Geometry: final body of the model. Coordinates: model frame, mm. Round coordinates to 2 decimals unless told otherwise and drop trailing zeros. Write each loop counter-clockwise with the first axis right and the second up, starting at its lowest first coordinate (ties: lowest second). Pieces come first, ordered by that corner, then holes. Notation, with made-up numbers: M -25,46 L -21,46 A18 ccw -21,54 Z; hole C -17,84.25 d1. An arc over 180 degrees is marked long. Use one line per item in the form item = value. Start each with the question number.
Item 1: Section query B-B (z = 31). Return loops of the section in (x, y).
Item 2: Ray query, probe 1 along X at (y, z) = (14, 29); probe 2 along Y at (x, z) = (131, 33); probe 3 along Y at (x, z) = (15, 29). Return the intervals inside material, ascending.
Item 3: Section query A-A (y = 15). Return loops of the section in (x, z).
Item 4: Pin query (flat end, axial travel): pin 1 Ø5 at (x, y) = (105, 76) entering from -Z; pin 2 Ø7 at (x, y) = (185, 15) entering from -Z; pin 3 Ø3 at (x, z) = (133.5, 22) entering from +Y; pin 4 Ø1 at (x, z) = (42, 5.5) entering from +Y. Return the tip coordinate at first contact, or that it passes through.
from build123d import *

# Parameters (mm, degrees)
F1_DEPTH = 50
F2_R     = 5
F3_R     = 4
F4_DEPTH = 50.001


with BuildPart() as f1:
    # F0 (on Top) → F1 (new body)
    with BuildSketch(Plane.XY):
        with BuildLine():
            Line((0, 57.2570811482), (0, 0))
            Line((0, 0), (200, 0))
            Line((200, 0), (200, 57.2570811482))
            ThreePointArc((200, 57.2570811482), (199.3836985076, 59.6619070036), (197.6867250421, 61.4738937535))
            Line((197.6867250421, 61.4738937535), (138.4492468932, 99.2168126053))
            ThreePointArc((138.4492468932, 99.2168126053), (137.1617961225, 99.8002116113), (135.7625218511, 100))
            Line((135.7625218511, 100), (129.5803989155, 100))
            ThreePointArc((129.5803989155, 100), (126.3529127937, 101.1811869209), (124.6503324296, 104.1666666667))
            ThreePointArc((124.6503324296, 104.1666666667), (100, 125), (75.3496675704, 104.1666666667))
            ThreePointArc((75.3496675704, 104.1666666667), (73.6470872063, 101.1811869209), (70.4196010845, 100))
            Line((70.4196010845, 100), (64.2374781489, 100))
            ThreePointArc((64.2374781489, 100), (62.8382038775, 99.8002116113), (61.5507531068, 99.2168126053))
            Line((61.5507531068, 99.2168126053), (2.3132749579, 61.4738937535))
            ThreePointArc((2.3132749579, 61.4738937535), (0.6163014924, 59.6619070036), (0, 57.2570811482))
        make_face()
    extrude(amount=F1_DEPTH)

    # F2
    f2_edges = [f1.edges().sort_by_distance(p)[0] for p in [
        (0, 28.628541, 50),
        (100, 0, 50),
        (200, 28.628541, 50),
        (199.383699, 59.661907, 50),
        (168.067986, 80.345353, 50),
        (137.161796, 99.800212, 50),
        (132.67146, 100, 50),
        (126.352913, 101.181187, 50),
        (100, 125, 50),
        (73.647087, 101.181187, 50),
        (67.32854, 100, 50),
        (62.838204, 99.800212, 50),
        (31.932014, 80.345353, 50),
        (0.616301, 59.661907, 50),
    ]]
    fillet(f2_edges, radius=F2_R)

    # F3 (on face) → F4 (cut, through all)
    with BuildSketch(Plane.XY.offset(50)):
        with Locations((185, 15)):
            Circle(F3_R)
        with Locations((15, 15)):
            Circle(F3_R)
    extrude(amount=-F4_DEPTH, mode=Mode.SUBTRACT)


solid = f1.part
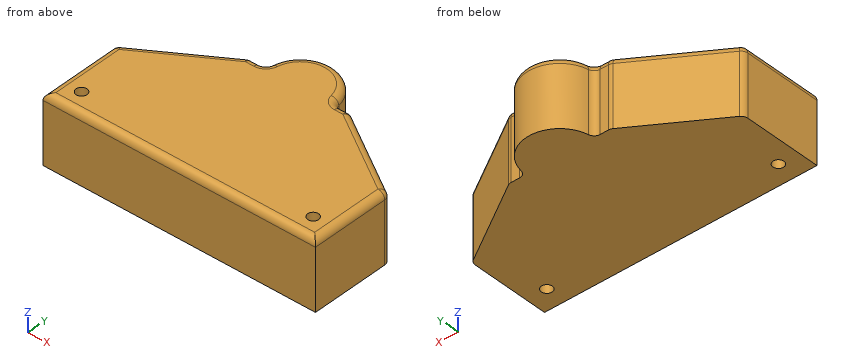
Working result:
q1.outline = M 0,0 L 200,0 L 200,57.26 A5 ccw 197.69,61.47 L 138.45,99.22 A5 ccw 135.76,100 L 129.58,100 A5 cw 124.65,104.17 A25 ccw 75.35,104.17 A5 cw 70.42,100 L 64.24,100 A5 ccw 61.55,99.22 L 2.31,61.47 A5 ccw 0,57.26 Z; hole C 15,15 d8; hole C 185,15 d8
q2.probe_1 = 0 to 11.13, 18.87 to 181.13, 188.87 to 200
q2.probe_2 = 0 to 100
q2.probe_3 = 0 to 11, 19 to 69.56
q3.outline = M 0,0 L 11,0 L 11,50 L 5,50 A5 ccw 0,45 Z; M 19,0 L 181,0 L 181,50 L 19,50 Z; M 189,0 L 200,0 L 200,45 A5 ccw 195,50 L 189,50 Z
q4.pin_1 = 0
q4.pin_2 = through
q4.pin_3 = 100
q4.pin_4 = 87.08
